Here's the drawing with two shaded views (mm, measured from the low corner). I have some questions. Round coordinates to 2 decimals unless told otherwise and drop trailing zeros. Loops run counter-clockwise (first coordinate to the right, second up) from the corner with the lowest first, then second, coordinate; pieces in that order, holes last. Notation, with made-up numbers: M 36.25,57 L 76.25,57 A11 ccw 76.25,76 Z; hole C 46.5,55.25 d6. An arc over 180 degrees is marked long. Answer as a JSON object with one key per item and string values.
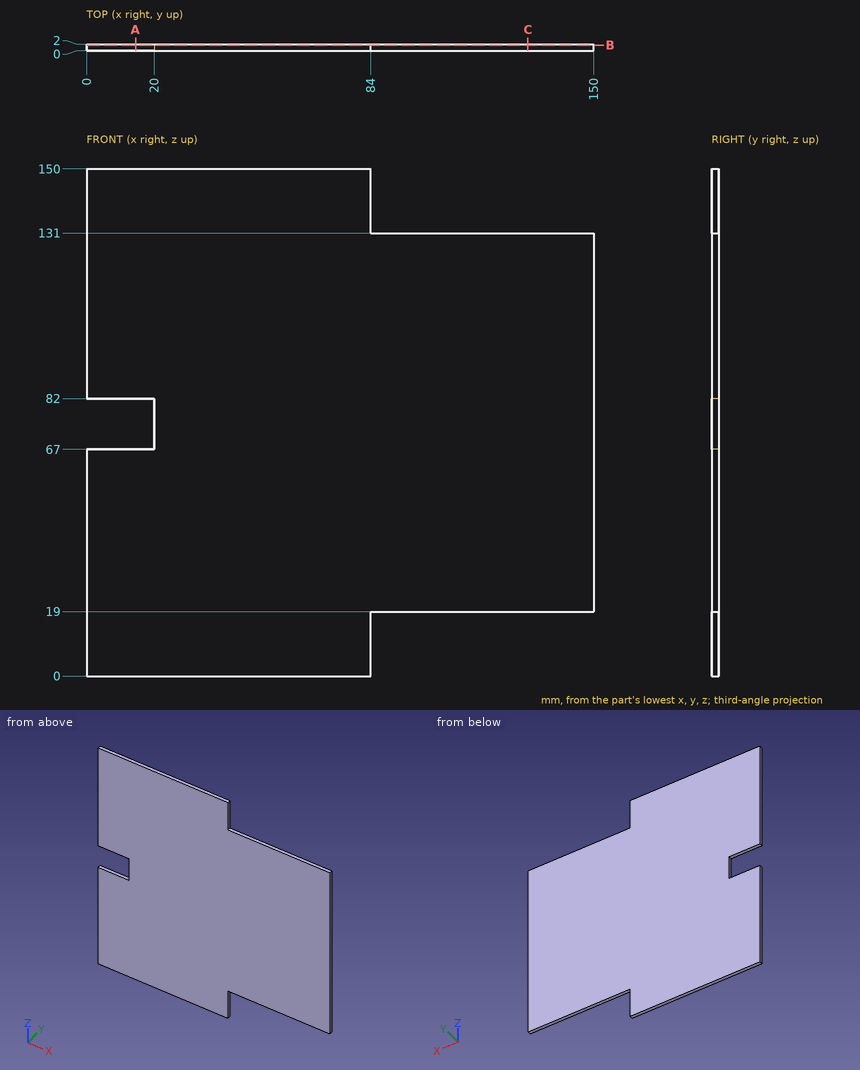
Item 1: For P1, Ø1, axis at x = 106.5, y = 1.5, coming from the -Z side; P2, Ø0.6, axis at y = 0.5, z = 72, coming from the -X side, each with a flat end and sliding along its axis, tell me the tip position at first contact or that it passes through.
Solution:
{"P1": "stops at z = 19", "P2": "stops at x = 20"}
Item 2: If I drill on L1, parallel to Z at x = 125, y = 0.9; L2, parallel to X at y = 1, z = 80.5; L3, parallel to X at y = 1.35, z = 9, over which ranges is the centre line in solid material (lowest first)? Write a range as from..to.
Solution:
{"L1": "z = 19..131", "L2": "x = 20..150", "L3": "x = 0..84"}
Item 3: I want a section at C-C on x = 130.5. List the corners of the cut face in (y, z) for me, plus the area to 3 significant figures.
Solution:
{"outline": "M 0,19 L 2,19 L 2,131 L 0,131 Z", "area": "224 mm2"}
Item 4: I want a section at B-B on y = 1.65. List the corners of the cut face in (x, z) for me, plus the area to 3 significant figures.
Solution:
{"outline": "M 0,0 L 84,0 L 84,19 L 150,19 L 150,131 L 84,131 L 84,150 L 0,150 L 0,82 L 20,82 L 20,67 L 0,67 Z", "area": "19,700 mm2"}
Item 5: I want a section at A-A on x = 14.5. List the corners of the cut face in (y, z) for me, plus the area to 3 significant figures.
Solution:
{"outline": "M 0,0 L 2,0 L 2,67 L 0,67 Z; M 0,82 L 2,82 L 2,150 L 0,150 Z", "area": "270 mm2"}
